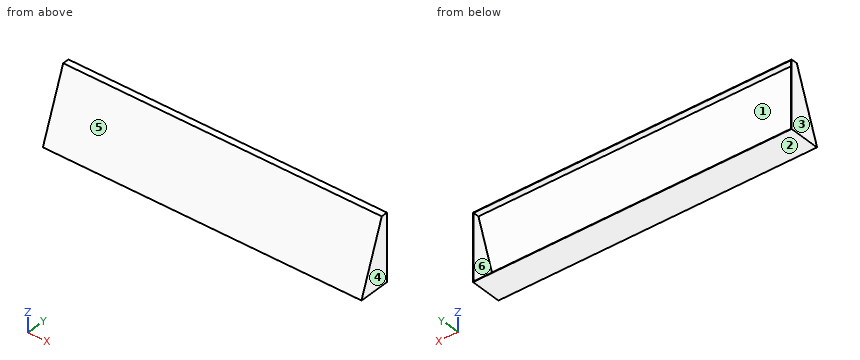
from build123d import *

# Parameters (mm, degrees)
SKETCH1_W           = 510
SKETCH1_H           = 50
BOSS_EXTRUDE1_DEPTH = 0.8
BOSS_EXTRUDE2_DEPTH = 510
SHELL3_T            = -0.8


with BuildPart() as part:
    # Sketch1 → Boss-Extrude1 (new body)
    with BuildSketch(Plane.XY):
        with Locations((255, 25)):
            Rectangle(SKETCH1_W, SKETCH1_H)
    extrude(amount=BOSS_EXTRUDE1_DEPTH)

    # Sketch3 → Boss-Extrude2 (add)
    with BuildSketch(Plane.ZY):
        Polygon((0.8, 0), (106.948846413, 39.715428922), (106.948846413, 50), (90.052783597, 50), (89.601213207, 50), (74.506616927, 50), (0.8, 50), align=None)
    extrude(amount=-BOSS_EXTRUDE2_DEPTH)

    # Shell3
    shell3_openings = [part.faces().sort_by_distance(p)[0] for p in [
        (255, 50, 53.474423206),
    ]]
    offset(amount=SHELL3_T, openings=shell3_openings, kind=Kind.INTERSECTION)


solid = part.part
The model under review builds one solid part; all positions refer to its coordinate system, in mm. Face numbers are marked on the shaded views. A direction names the side the tool comes from. Round coordinates to 2 decimals unless told otherwise and drop trailing zeros. Loops run counter-clockwise (first coordinate to the right, second up) from the corner with the lowest first, then second, coordinate; pieces in that order, holes last. Notation, with made-up numbers: (-23, 12.5) -> (-14, 12.5) arc R19 ccw to (-14, 27.5) -> close; hole circle Ø5 at (48, 30.25). An arc over 180 degrees is marked (long way). Return JSON: item names as keys, results as strings.
(1) For line 1 (X direction, y = 31.5, z = 61.5); line 2 (Z direction, x = 488, y = 41); line 3 (Y direction, x = 58.5, z = 93.5), list the stretches that pass through material, from the lowest coordinate up.
Solved:
{"line 1": "0 to 0.8, 509.2 to 510", "line 2": "0 to 0.8, 106.15 to 106.95", "line 3": "34.68 to 35.54"}
(2) Add section D-D on z = 68.5. Write out the cut boundary in (x, y), plus the area to 3 significant figures.
Solved:
{"outline": "(0, 25.33) -> (510, 25.33) -> (510, 50) -> (509.2, 50) -> (509.2, 26.18) -> (0.8, 26.18) -> (0.8, 50) -> (0, 50) -> close", "area": "474 mm2"}
(3) Add section A-A on y = 20. Write out the cut boundary in (x, z).
Solved:
{"outline": "(0, 0) -> (510, 0) -> (510, 54.25) -> (0, 54.25) -> close; hole (0.8, 0.8) -> (509.2, 0.8) -> (509.2, 51.97) -> (0.8, 51.97) -> close"}
(4) The part is to be moulded in two halves that separate along X. For the marked faces 1, 2, 3 and 4, say which applies: released by +X, released by -X, zero draft, split by the parting line, or undercut.
Solved:
{"face 1": "undercut", "face 2": "zero draft", "face 3": "released by -X", "face 4": "released by +X"}
(5) For the marked faces 5 and 6, list the 3-axis set-ups (+Z, -Z, +X, -X, +Y, -Y) from which the entire face can be reached by the end or side of a thin tool; tool diameter is ignored.
Solved:
{"face 5": "+Z, +X, -X, -Y", "face 6": "+Y"}
(6) For pin 1 (1 mm diameter, centred on x = 236.5, z = 49, fed in from -Y); pin 2 (12 mm diameter, centred on x = 347.5, y = 42.5, fed in from -Z); pin 3 (6 mm diameter, centred on x = 434.5, z = 90.5, fed in from -Y); pin 4 (1 mm diameter, centred on x = 234.5, z = 39, fed in from -Y), all flat-tipped, find the tip position at first contact; note any pin that passes through.
Solved:
{"pin 1": "y = 17.85", "pin 2": "z = 0", "pin 3": "y = 32.44", "pin 4": "y = 14.11"}
(7) Add section B-B on x = 330.5. Write out the cut boundary in (y, z), plus the area to 3 significant figures.
Solved:
{"outline": "(0, 0) -> (50, 0) -> (50, 0.8) -> (0.85, 0.8) -> (40.27, 106.15) -> (50, 106.15) -> (50, 106.95) -> (39.72, 106.95) -> (0, 0.8) -> close", "area": "138 mm2"}
(8) Add section C-C on z = 22.5. Write out the cut boundary in (x, y).
Solved:
{"outline": "(0, 8.12) -> (510, 8.12) -> (510, 50) -> (509.2, 50) -> (509.2, 8.97) -> (0.8, 8.97) -> (0.8, 50) -> (0, 50) -> close"}
